Here's how the part is built. I have some questions about the finished solid (model axes, mm). A direction names the side the tool comes from. Round coordinates to 2 decimals unless told otherwise and drop trailing zeros. Write each loop counter-clockwise with the first axis right and the second up, starting at its lowest first coordinate (ties: lowest second). Pieces come first, ordered by that corner, then holes. Notation, with made-up numbers: (32, 75.25) -> (37, 75.25) arc R4 ccw to (37, 81.25) -> close; hole circle Ø2 at (6.25, 72). An arc over 180 degrees is marked (long way). Put each result on its own line as item: value. Start each with the question number.
1. Suppose I cut it at C-C (x = -15.5). Please give me the cut outline in (y, z), then the cut area to 3 significant figures.
2. For pin 1 (2.5 mm diameter, centred on x = -15, z = -15, fed in from +Y); pin 2 (1.5 mm diameter, centred on x = 16, z = 16, fed in from +Y); pin 3 (10 mm diameter, centred on x = 3, z = 11, fed in from +Y), each with a flat end and sliding along its axis, tell me the tip position at first contact or that it passes through.
3. Which directions (+Z, -Z, +X, -X, +Y, -Y) give clear straight access to the entire face, cutting with the end or side of a thin tool? Please do faces 4 (the face through (0, 10, -21.15)), 5 (the face through (15, 18, 15)).
4. Suppose I cut it at D-D (y = 31). Please give me the cut outline in (x, z), then the cut area to 3 significant figures.
5. Suppose I cut it at A-A (z = 15.5). Please give me the cut outline in (x, y).
6. I need wall thicknesses on probe 1 along X at (y, z) = (19, -15.5); probe 2 along Y at (x, z) = (8, 8); probe 3 along Z at (x, y) = (-1, 30). Which ranges of each line are inside material? Lowest first, please. Write a range as from..to.
7. Suppose I cut it at B-B (y = 13). Please give me the cut outline in (x, z).
8. We'd pull the mould along X, two halves only. Please class faces 1 (the face through (14, 19.52, 15.43)), 2 (the face through (21.15, 10, 0)), 3 (the face through (-18.6, 10.4, -18.7)): +X half, -X half, draft (parallel to the pull), parting line (faces both ways), or undercut.
```python
from build123d import *

# Parameters (mm, degrees)
SKETCH1_W           = 42.3
SKETCH1_H           = 42.3
BOSS_EXTRUDE1_DEPTH = 21
CHAMFER1_SIZE       = 5
SKETCH2_R           = 1.5
CUT_EXTRUDE1_DEPTH  = 3
SKETCH3_R           = 11
BOSS_EXTRUDE2_DEPTH = 2
SKETCH4_R           = 2.5
BOSS_EXTRUDE3_DEPTH = 15


with BuildPart() as part:
    # Sketch1 → Boss-Extrude1 (new body)
    with BuildSketch(Plane(origin=(0, 0, 0), x_dir=(1, 0, 0), z_dir=(0, 1, 0))):
        Rectangle(SKETCH1_W, SKETCH1_H)
    extrude(amount=BOSS_EXTRUDE1_DEPTH)

    # Chamfer1
    chamfer1_edges = [part.edges().sort_by_distance(p)[0] for p in [
        (21.15, 10.5, 21.15),
        (-21.15, 10.5, 21.15),
        (-21.15, 10.5, -21.15),
        (21.15, 10.5, -21.15),
    ]]
    chamfer(chamfer1_edges, length=CHAMFER1_SIZE)

    # Sketch2 → Cut-Extrude1 (cut)
    with BuildSketch(Plane(origin=(0, 21, 0), x_dir=(1, 0, 0), z_dir=(0, 1, 0))):
        with Locations((15.5, -15.5)):
            Circle(SKETCH2_R)
        with Locations((15.5, 15.5)):
            Circle(SKETCH2_R)
        with Locations((-15.5, 15.5)):
            Circle(SKETCH2_R)
        with Locations((-15.5, -15.5)):
            Circle(SKETCH2_R)
    extrude(amount=-CUT_EXTRUDE1_DEPTH, mode=Mode.SUBTRACT)

    # Sketch3 → Boss-Extrude2 (add)
    with BuildSketch(Plane(origin=(0, 21, 0), x_dir=(1, 0, 0), z_dir=(0, 1, 0))):
        Circle(SKETCH3_R)
    extrude(amount=BOSS_EXTRUDE2_DEPTH)

    # Sketch4 → Boss-Extrude3 (add)
    with BuildSketch(Plane(origin=(0, 23, 0), x_dir=(1, 0, 0), z_dir=(0, 1, 0))):
        Circle(SKETCH4_R)
    extrude(amount=BOSS_EXTRUDE3_DEPTH)


solid = part.part
```
Verdict:
1. outline: (0, -21.15) -> (21, -21.15) -> (21, -17) -> (18, -17) -> (18, -14) -> (21, -14) -> (21, 14) -> (18, 14) -> (18, 17) -> (21, 17) -> (21, 21.15) -> (0, 21.15) -> close
1. area: 870 mm^2
2. pin 1: stops at y = 21
2. pin 2: stops at y = 18
2. pin 3: stops at y = 23
3. face 4: -Z, +X, -X, +Y, -Y
3. face 5: +Y
4. outline: circle Ø5 at (0, 0)
4. area: 19.6 mm^2
5. outline: (-21.15, 0) -> (21.15, 0) -> (21.15, 21) -> (17, 21) -> (17, 18) -> (14, 18) -> (14, 21) -> (-14, 21) -> (-14, 18) -> (-17, 18) -> (-17, 21) -> (-21.15, 21) -> close
6. probe 1: x = -21.15..-17, -14..14, 17..21.15
6. probe 2: y = 0..21
6. probe 3: z = -2.29..2.29
7. outline: (-21.15, -16.15) -> (-16.15, -21.15) -> (16.15, -21.15) -> (21.15, -16.15) -> (21.15, 16.15) -> (16.15, 21.15) -> (-16.15, 21.15) -> (-21.15, 16.15) -> close
8. face 1: undercut
8. face 2: +X half
8. face 3: -X half
